Source: three-view drawing plus pictorial views. Frame: mm from the lowest corner of the part. A direction names the side the tool comes from. Give positions to 0.01 mm unless a question says otherwise; leave off trailing zeros. Loops run counter-clockwise (first coordinate to the right, second up) from the corner with the lowest first, then second, coordinate; pieces in that order, holes last. Notation, with made-up numbers: (56.5, 47) - (66.5, 47) arc R17 ccw to (66.5, 57) - close; hole circle Ø7 at (18, 18). An arc over 180 degrees is marked (long way). Write each question's results on one line, items separated by ' | '. Start each with the question number.
(1) Cut plane A-A on z = 15. Return the cut outline in (x, y).
(2) Cut plane C-C on y = 6.5. Return the cut outline in (x, z), then the cut area to 3 significant figures.
(3) Cut plane D-D on x = 5. Return the cut outline in (y, z).
(4) Cut plane B-B on y = 28. Return the cut outline in (x, z).
(5) Contact query for flat-ended pins moving along their axis: pin 1 (2 mm diameter, centred on x = 9, z = 14, fed in from -Y); pin 2 (9.5 mm diameter, centred on x = 22, z = 15, fed in from -Y); pin 3 (3 mm diameter, centred on x = 4.5, y = 20, fed in from +Z); pin 4 (12 mm diameter, centred on x = 5.5, y = 32, fed in from +Z) (3 decimals). Output: stop coordinate, or through.
(6) Pull-direction query (X, two-part tool) for the marked faces 1, 2, 3 and 4; classes: pulls with the +X half, pulls with the -X half, needs draft (parallel to the pull), parting line crosses it, or undercut.
(7) Reachability of the marked faces 5, 6 and 7 from +Z, -Z, +X, -X, +Y, -Y: full face, straight path, thin tool, end or side. Return the list, or none.
(8) Material intervals for line 1 along Y through (x, z) = (39, 14.5); line 2 along X through (y, z) = (6, 16); line 3 along Y through (x, z) = (6, 22), sorted ascending. Write a range as [from, to].
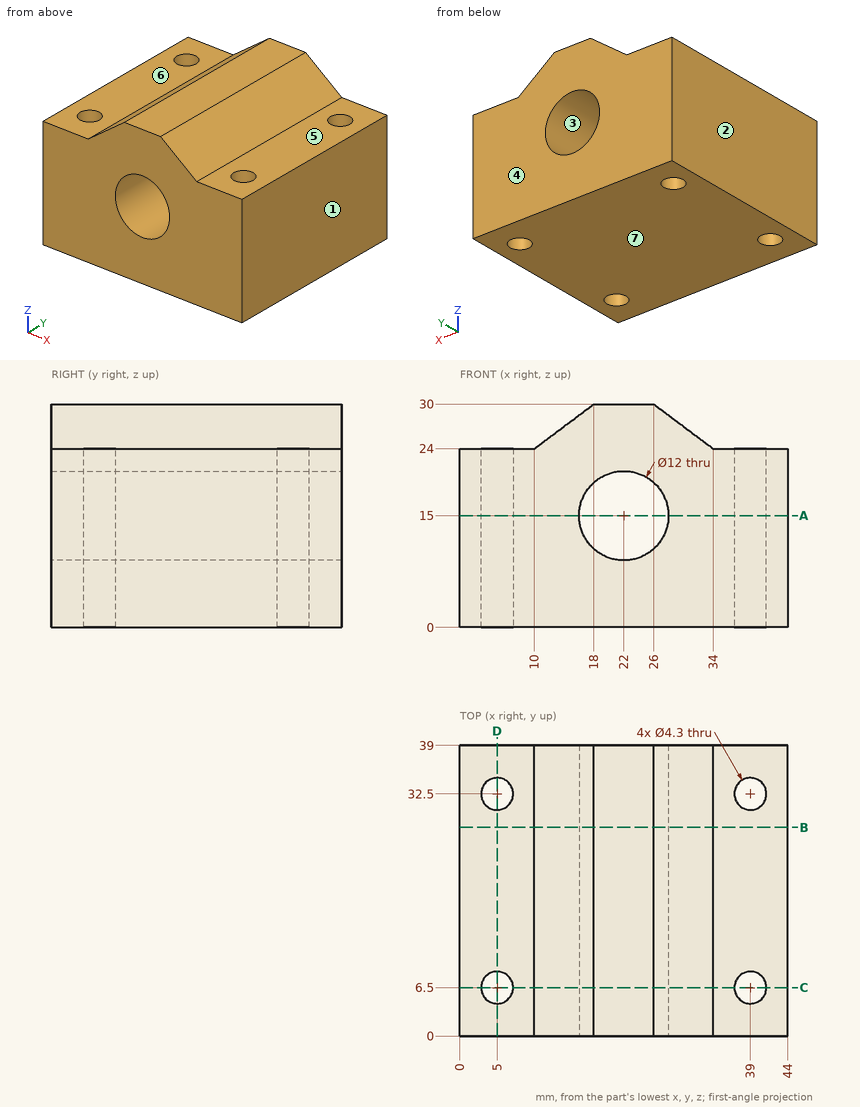
Ans:
1) outline: (0, 0) - (16, 0) - (16, 39) - (0, 39) - close; (28, 0) - (44, 0) - (44, 39) - (28, 39) - close; hole circle Ø4.3 at (5, 6.5); hole circle Ø4.3 at (5, 32.5); hole circle Ø4.3 at (39, 6.5); hole circle Ø4.3 at (39, 32.5)
2) outline: (0, 0) - (2.85, 0) - (2.85, 24) - (0, 24) - close; (7.15, 0) - (36.85, 0) - (36.85, 24) - (34, 24) - (26, 30) - (18, 30) - (10, 24) - (7.15, 24) - close; (41.15, 0) - (44, 0) - (44, 24) - (41.15, 24) - close; hole circle Ø12 at (22, 15) | area: 833 mm^2
3) outline: (0, 0) - (4.35, 0) - (4.35, 24) - (0, 24) - close; (8.65, 0) - (30.35, 0) - (30.35, 24) - (8.65, 24) - close; (34.65, 0) - (39, 0) - (39, 24) - (34.65, 24) - close
4) outline: (0, 0) - (44, 0) - (44, 24) - (34, 24) - (26, 30) - (18, 30) - (10, 24) - (0, 24) - close; hole circle Ø12 at (22, 15)
5) pin 1: y = 0 | pin 2: through | pin 3: z = 24 | pin 4: z = 25.125
6) face 1: pulls with the +X half | face 2: pulls with the -X half | face 3: undercut | face 4: needs draft
7) face 5: +Z, +X, +Y, -Y | face 6: +Z, -X, +Y, -Y | face 7: -Z, +X, -X, +Y, -Y
8) line 1: [0, 4.35], [8.65, 30.35], [34.65, 39] | line 2: [0, 2.91], [7.09, 16.08], [27.92, 36.91], [41.09, 44] | line 3: [0, 4.6], [8.4, 30.6], [34.4, 39]
